from build123d import *

# Parameters (mm, degrees)
EXTRUDE_1_DEPTH     = 38
SKETCH_2_R          = 11
EXTRUDE_2_DEPTH     = 2
SKETCH_3_R          = 2.5
EXTRUDE_3_DEPTH     = 21.5
CUT_EXTRUDE_1_REACH = 80.461
SKETCH_4_R          = 1.5


with BuildPart() as part:
    # 草图1 → 凸台-拉伸1 (new body)
    with BuildSketch(Plane.XY):
        Polygon((-39.221447105, 9.245047294), (-35.071447105, 13.395047294), (-1.071447105, 13.395047294), (3.078552895, 9.245047294), (3.078552895, -24.754952706), (-1.071447105, -28.904952706), (-35.071447105, -28.904952706), (-39.221447105, -24.754952706), align=None)
    extrude(amount=EXTRUDE_1_DEPTH)

    # 草图2 → 凸台-拉伸2 (add)
    with BuildSketch(Plane.XY.offset(38)):
        with Locations((-18.071447105, -7.754952706)):
            Circle(SKETCH_2_R)
    extrude(amount=EXTRUDE_2_DEPTH)

    # 草图3 → 凸台-拉伸3 (add)
    with BuildSketch(Plane.XY.offset(40)):
        with Locations((-18.071447105, -7.754952706)):
            Circle(SKETCH_3_R)
    extrude(amount=EXTRUDE_3_DEPTH)

    # 草图4 → 切除-拉伸1 (cut, up to next)
    with BuildSketch(Plane(origin=(0, 0, 0), x_dir=(-1, 0, 0), z_dir=(0, 0, -1)), mode=Mode.PRIVATE) as cut_extrude_1_sk1:
        with Locations((2.571447105, 7.745047294)):
            Circle(SKETCH_4_R)
    cut_extrude_1_tool1 = extrude(cut_extrude_1_sk1.sketch, amount=-CUT_EXTRUDE_1_REACH, mode=Mode.PRIVATE) & part.part
    # 草图4 → 切除-拉伸1 (cut, up to next)
    with BuildSketch(Plane(origin=(0, 0, 0), x_dir=(-1, 0, 0), z_dir=(0, 0, -1)), mode=Mode.PRIVATE) as cut_extrude_1_sk2:
        with Locations((2.571447105, -23.254952706)):
            Circle(SKETCH_4_R)
    cut_extrude_1_tool2 = extrude(cut_extrude_1_sk2.sketch, amount=-CUT_EXTRUDE_1_REACH, mode=Mode.PRIVATE) & part.part
    # 草图4 → 切除-拉伸1 (cut, up to next)
    with BuildSketch(Plane(origin=(0, 0, 0), x_dir=(-1, 0, 0), z_dir=(0, 0, -1)), mode=Mode.PRIVATE) as cut_extrude_1_sk3:
        with Locations((33.571447105, -23.254952706)):
            Circle(SKETCH_4_R)
    cut_extrude_1_tool3 = extrude(cut_extrude_1_sk3.sketch, amount=-CUT_EXTRUDE_1_REACH, mode=Mode.PRIVATE) & part.part
    # 草图4 → 切除-拉伸1 (cut, up to next)
    with BuildSketch(Plane(origin=(0, 0, 0), x_dir=(-1, 0, 0), z_dir=(0, 0, -1)), mode=Mode.PRIVATE) as cut_extrude_1_sk4:
        with Locations((33.571447105, 7.745047294)):
            Circle(SKETCH_4_R)
    cut_extrude_1_tool4 = extrude(cut_extrude_1_sk4.sketch, amount=-CUT_EXTRUDE_1_REACH, mode=Mode.PRIVATE) & part.part
    add(cut_extrude_1_tool1.solids().sort_by_distance((-2.571447, 7.745047, 0))[0], mode=Mode.SUBTRACT)
    add(cut_extrude_1_tool2.solids().sort_by_distance((-2.571447, -23.254953, 0))[0], mode=Mode.SUBTRACT)
    add(cut_extrude_1_tool3.solids().sort_by_distance((-33.571447, -23.254953, 0))[0], mode=Mode.SUBTRACT)
    add(cut_extrude_1_tool4.solids().sort_by_distance((-33.571447, 7.745047, 0))[0], mode=Mode.SUBTRACT)


solid = part.part
Can you work these out from the model? Positions are in its coordinate system, mm. A direction names the side the tool comes from. Coordinates: 2 decimals unless noted, no trailing zeros. Loops run counter-clockwise (first coordinate to the right, second up) from the corner with the lowest first, then second, coordinate; pieces in that order, holes last. Notation, with made-up numbers: (43, 75.5) - (96, 75.5) arc R24 cw to (96, 110.5) - close; hole circle Ø7 at (50, 25). An arc over 180 degrees is marked (long way). Answer as a JSON object with one key per item and string values. Group by question number.
Item 1: If we section it at C-C (x = -8): List the corners of the cut face in (y, z) for me, plus the area to 3 significant figures.
Item 2: If we mould it in two halves opening along X, with no side actions, what happens to faces 1 (the face through (-33.376, 9.232, 18.734)), 2 (the face through (-2.25, -24.72, 18.73)), 3 (the face through (-18, -28.905, 19)), 4 (the face through (-37.175, 11.291, 18.734))? For each: released by +X, released by -X, zero draft, split by the parting line, or undercut.
Item 3: If we section it at A-A (y = 7): List the corners of the cut face in (x, z) for me.
Item 4: If I drill on L1, parallel to Y at x = -33.5, z = 23.5; L2, parallel to Z at x = -9, y = 2; L3, parallel to Z at x = -20, y = -4.5, over which ranges is the centre line in solid material (lowest first)? Write a range as from..to.
Item 5: On a 3-axis mill with a long thin cutter (end or side, diameter ignored), from which of +Z, -Z, +X, -X, +Y, -Y can I reach the whole of each face in a straight line? I mean faces 5 (the face through (-33.25, -24.72, 18.73)), 6 (the face through (-27, -17, 38)). Say none if no direction works.
Item 6: If we section it at B-B (z = 14.5): List the corners of the cut face in (x, y) for me, plus the area to 3 significant figures.
Item 7: For pin 1 (4 mm diameter, centred on x = -33.57, y = 7.75, fed in from +Z); pin 2 (3 mm diameter, centred on x = -29, z = 43, fed in from -Y), each with a flat end and sliding along its axis, tell me the tip position at first contact or that it passes through.
Item 8: If we section it at D-D (y = -7): List the corners of the cut face in (x, z) for me.
Returned:
{
 "1": {"outline": "(-28.9, 0) - (13.4, 0) - (13.4, 38) - (-3.33, 38) - (-3.33, 40) - (-12.18, 40) - (-12.18, 38) - (-28.9, 38) - close", "area": "1,630 mm²"},
 "2": {"face 1": "undercut", "face 2": "undercut", "face 3": "zero draft", "face 4": "released by -X"},
 "3": {"outline": "(-39.22, 0) - (-34.87, 0) - (-34.87, 38) - (-39.22, 38) - close; (-32.27, 0) - (-3.87, 0) - (-3.87, 38) - (-32.27, 38) - close; (-1.27, 0) - (3.08, 0) - (3.08, 38) - (-1.27, 38) - close"},
 "4": {"L1": "y = -28.9..-24.75, -21.76..6.25, 9.24..13.4", "L2": "z = 0..38", "L3": "z = 0..40"},
 "5": {"face 5": "+Z, -Z", "face 6": "+Z"},
 "6": {"outline": "(-39.22, -24.75) - (-35.07, -28.9) - (-1.07, -28.9) - (3.08, -24.75) - (3.08, 9.25) - (-1.07, 13.4) - (-35.07, 13.4) - (-39.22, 9.25) - close; hole circle Ø3 at (-33.57, -23.25); hole circle Ø3 at (-33.57, 7.75); hole circle Ø3 at (-2.57, -23.25); hole circle Ø3 at (-2.57, 7.75)", "area": "1,730 mm²"},
 "7": {"pin 1": "stops at z = 38", "pin 2": "passes through"},
 "8": {"outline": "(-39.22, 0) - (3.08, 0) - (3.08, 38) - (-7.1, 38) - (-7.1, 40) - (-15.69, 40) - (-15.69, 61.5) - (-20.45, 61.5) - (-20.45, 40) - (-29.05, 40) - (-29.05, 38) - (-39.22, 38) - close"}
}
